Autodesk Inventor part; units mm, degrees
ref_plane "YZ Plane" through (0, 0, 0) normal (1, 0, 0) x (0, 1, 0)
ref_plane "XZ Plane" through (0, 0, 0) normal (0, 1, 0) x (-1, 0, 0)
ref_plane "XY Plane" through (0, 0, 0) normal (0, 0, 1) x (1, 0, 0)
sketch "Esquisse1" plane through (0, 0, 0) normal (0, 0, 1) x (1, 0, 0)
  line L0 (0, 0) -> (98.8, 0)
  line L1 (98.8, 0) -> (98.8, 49.4)
  line L2 (98.8, 49.4) -> (0, 49.4)
  line L3 (0, 49.4) -> (0, 0)
  dimension "d0" = 98.8
  dimension "d1" = 49.4
extrude "Extrusion1" add sketch "Esquisse1" along normal blind 5
sketch "Esquisse2" plane through (98.8, 0, 0) normal (1, 0, 0) x (0, 0, -1)
  line L0 (0, 49.4) -> (-5, 49.4)
  line L1 (-5, 49.4) -> (-66.3, 49.4)
  line L2 (-84.3, 31.4) -> (-84.3, 18)
  line L3 (-66.3, 0) -> (-5, 0)
  line L4 (-5, 0) -> (-5, 49.4)
  arc A0 (-66.3, 49.4) -> (-84.3, 31.4) centre (-66.3, 31.4) ccw
  arc A1 (-84.3, 18) -> (-66.3, 0) centre (-66.3, 18) ccw
  point P0 (0, 0)
  point P1 (-84.3, 49.4)
  dimension "d4" = 79.3
  dimension "d5" = 49.4
  dimension "d6" = 18
  dimension "d7" = 18
extrude "Extrusion2" add sketch "Esquisse2" against normal blind 5
sketch "Esquisse3" plane through (0, 0, 0) normal (-1, 0, 0) x (0, 0, 1)
  line L0 (66.3, 49.4) -> (5, 49.4)
  line L1 (5, 49.4) -> (66.3, 49.4)
  line L2 (84.3, 31.4) -> (84.3, 18)
  line L3 (66.3, 0) -> (5, 0)
  line L4 (5, 0) -> (5, 49.4)
  arc A0 (66.3, 0) -> (84.3, 18) centre (66.3, 18) ccw
  arc A1 (84.3, 31.4) -> (66.3, 49.4) centre (66.3, 31.4) ccw
  point P0 (0, 0)
  point P1 (84.3, 0)
  dimension "d13" = 79.3
  dimension "d14" = 49.4
  dimension "d15" = 18
extrude "Extrusion3" add sketch "Esquisse3" against normal blind 5
sketch "Esquisse4" plane through (0, 0, 0) normal (-1, 0, 0) x (0, 0, 1)
  circle A0 centre (64.8, 24.7) radius 5
  line L0 (84.3, 31.4) -> (84.3, 18)
  line L1 (0, 0) -> (66.3, 0)
  dimension "d18" = 10
  dimension "d19" = 19.5
  dimension "d20" = 24.7
extrude "Extrusion4" cut sketch "Esquisse4" against normal blind 5
sketch "Esquisse5" plane through (98.8, 0, 0) normal (1, 0, 0) x (0, 0, -1)
  circle A0 centre (-64.8, 24.7) radius 5
  line L0 (0, 49.4) -> (-66.3, 49.4)
  line L1 (-84.3, 31.4) -> (-84.3, 18)
  point P0 (0, 0)
  dimension "d23" = 10
  dimension "d24" = 24.7
  dimension "d25" = 19.5
extrude "Extrusion5" cut sketch "Esquisse5" against normal blind 5
sketch "Esquisse6" plane through (0, 0, 0) normal (0, 0, -1) x (-1, 0, 0)
  line L0 (-98.8, 49.4) -> (0, 49.4)
  line L1 (0, 0) -> (-98.8, 49.4)
  line L2 (-98.8, 0) -> (-98.8, 49.4)
  line L3 (-98.8, 0) -> (0, 49.4)
  circle A0 centre (-49.4, 24.7) radius 5
  dimension "d28" = 10
extrude "Extrusion6" cut sketch "Esquisse6" against normal blind 5 contours A0 L3 L1 | L1 L3 A0 | A0 L1 L3 | L1 A0 L3
fillet "Congé1" radius 2 2 edges at (93.8, 24.7, 5) (5, 24.7, 5)
properties part number "ShoulderPart2" material "Plastique ABS"
Model file for the job. Use its own axes, mm. A direction names the side the tool comes from. Round coordinates to 2 decimals unless told otherwise and drop trailing zeros. Write each loop counter-clockwise with the first axis right and the second up, starting at its lowest first coordinate (ties: lowest second). Pieces come first, ordered by that corner, then holes. Notation, with made-up numbers: M 45,-4 L 53,-4 A10 ccw 53,2 Z; hole C 77,69 d10. An arc over 180 degrees is marked long. Put each result on its own line as item: value.
Item 1: Probe L1, parallel to X at y = 15.5, z = 51; L2, parallel to Y at x = 95.25, z = 64.8; L3, parallel to Z at x = 37, y = 30.5. List the from-to ranges inside material, lowest first. Write a range as from..to.
Responses:
L1: 0..5, 93.8..98.8
L2: 0..19.7, 29.7..49.4
L3: 0..5
Item 2: Cut at B-B (z = 64.8). List the corners of the cut face in (x, y).
Responses:
outline: M 0,0 L 5,0 L 5,19.7 L 0,19.7 Z; M 0,29.7 L 5,29.7 L 5,49.4 L 0,49.4 Z; M 93.8,0 L 98.8,0 L 98.8,19.7 L 93.8,19.7 Z; M 93.8,29.7 L 98.8,29.7 L 98.8,49.4 L 93.8,49.4 Z
Item 3: Cut at A-A (y = 24.7). List the corners of the cut face in (x, z), and give its area (3 significant figures).
Responses:
outline: M 0,0 L 44.4,0 L 44.4,5 L 7,5 A2 cw 5,7 L 5,59.8 L 0,59.8 Z; M 0,69.8 L 5,69.8 L 5,84.3 L 0,84.3 Z; M 54.4,0 L 98.8,0 L 98.8,59.8 L 93.8,59.8 L 93.8,7 A2 cw 91.8,5 L 54.4,5 Z; M 93.8,69.8 L 98.8,69.8 L 98.8,84.3 L 93.8,84.3 Z
area: 1,140 mm²
Item 4: Tool access for faces 1 (the flat face through (49, 31, 5)), 2 (the cylindrical face through (96.335, 44.267, 78.887)): list every direction of +Z, -Z, +X, -X, +Y, -Y with a clear straight run to the whole face (end or side of a thin tool).
Responses:
face 1: +Z, +Y, -Y
face 2: +Z, +X, -X, +Y
Item 5: Cut at C-C (x = 49.4). List the corners of the cut face in (y, z).
Responses:
outline: M 0,0 L 19.7,0 L 19.7,5 L 0,5 Z; M 29.7,0 L 49.4,0 L 49.4,5 L 29.7,5 Z
Item 6: Mould opens along X. For faces 3 (the flat face through (49, 49.4, 4)), 4 (the flat face through (98.8, 24, 42)), 5 (the flat face through (93.8, 25, 46)), 6 (the flat face through (0, 25, 42)) say: +X half, -X half, draft (parallel to the pull), parting line (faces both ways), or undercut.
Responses:
face 3: draft
face 4: +X half
face 5: undercut
face 6: -X half
Item 7: Cut at D-D (z = 30). List the corners of the cut face in (x, y).
Responses:
outline: M 0,0 L 5,0 L 5,49.4 L 0,49.4 Z; M 93.8,0 L 98.8,0 L 98.8,49.4 L 93.8,49.4 Z
Item 8: Flat gauge pins, fed straight in: P1, Ø8, axis at x = 49.4, y = 24.7, coming from the +Z side; P2, Ø4, axis at x = 41, y = 23.5, coming from the +Z side. Where does each tip first touch, or does it go through?
Responses:
P1: through
P2: z = 5
